The listing builds one solid part. Answer for the finished solid, in the listing's coordinates (mm). Face numbers are marked on the shaded views. A direction names the side the tool comes from. Round coordinates to 2 decimals unless told otherwise and drop trailing zeros. Write each loop counter-clockwise with the first axis right and the second up, starting at its lowest first coordinate (ties: lowest second). Pieces come first, ordered by that corner, then holes.
(1) The mould has two halves that part along Y. Classify the marked faces 1, 2 and 3: +Y half, -Y half, draft (parallel to the pull), parting line (faces both ways), or undercut.
(2) For the marked faces 4, 5, 6, 7 and 8, determine the directions among +Z, -Z, +X, -X, +Y, -Y from which every point of the face is accessible in a straight line to the end or side of a thin tool.
(3) A cutting plane is placed at A-A, the plane y = 46.2. Give the vertices of the cut face in (x, z).
(4) A cutting plane is placed at B-B, the plane y = 12. Give the vertices of the cut face in (x, z).
(5) A cutting plane is placed at C-C, the plane x = 38.5. Give the vertices of the cut face in (y, z), and give its area (3 significant figures).
(6) Find the intervals of material crossed by probe 1 along Y at (x, z) = (34.3, 1.2); probe 2 along Y at (x, z) = (34.5, 15.25); probe 3 along X at (y, z) = (2.5, 5.75), in increasing order.
(7) Each of these flat-tipped pins is pushed along its axis until it touches: pin 1 Ø3 at (y, z) = (30, 8.5) entering from -X; pin 2 Ø2 at (x, z) = (20.5, 9.5) entering from -Y; pin 3 Ø5.5 at (x, y) = (7, 29) entering from +Z. Where does it stop, or does it pass through?
(8) A cutting plane is placed at D-D, the plane y = -3.25. Give the vertices of the cut face in (x, z), and give its area (3 significant figures).
from build123d import *

# Parameters (mm, degrees)
F1_DEPTH = 20
F0_R     = 1.75
F2_DEPTH = 2
F3_DEPTH = 1.3
F4_W     = 13.5
F4_H     = 6.9375
F4_H_2   = 1.25
F4_H_3   = 0.75
F5_DEPTH = 6.1
F6_DEPTH = 13.1
F7_R     = 3


with BuildPart() as f1:
    # F0 (on Top) → F1 (new body)
    with BuildSketch(Plane.XY):
        Polygon((15.3, 50), (15.3, 0), (25.3, 0), (43.3, 0), (53.3, 0), (53.3, 50), (43.3, 50), (25.3, 50), align=None)
    extrude(amount=F1_DEPTH)

    # F0 (on Top) → F2 (join)
    with BuildSketch(Plane.XY):
        with BuildLine():
            Line((43.3, 0), (25.3, 0))
            Line((25.3, 0), (32.379446801, -5.8995390008))
            ThreePointArc((32.379446801, -5.8995390008), (34.3, -6.594875162), (36.220553199, -5.8995390008))
            Line((36.220553199, -5.8995390008), (43.3, 0))
        make_face()
        with Locations((34.3, -3.25)):
            Circle(F0_R, mode=Mode.SUBTRACT)
        with BuildLine():
            Line((32.379446801, 55.8995390008), (25.3, 50))
            Line((25.3, 50), (43.3, 50))
            Line((43.3, 50), (36.220553199, 55.8995390008))
            ThreePointArc((36.220553199, 55.8995390008), (34.3, 56.594875162), (32.379446801, 55.8995390008))
        make_face()
        with Locations((34.3, 53.25)):
            Circle(F0_R, mode=Mode.SUBTRACT)
    extrude(amount=F2_DEPTH)

    # F0 (on Top) → F3 (join)
    with BuildSketch(Plane.XY):
        with BuildLine():
            ThreePointArc((0, 3), (0.8786796564, 0.8786796564), (3, 0))
            Line((3, 0), (15.3, 0))
            Line((15.3, 0), (15.3, 50))
            Line((15.3, 50), (3, 50))
            ThreePointArc((3, 50), (0.8786796564, 49.1213203436), (0, 47))
            Line((0, 47), (0, 3))
        make_face()
        with BuildLine():
            Line((11.0706789419, 2.3), (5.8, 2.3))
            ThreePointArc((5.8, 2.3), (4.3, 3.8), (5.8, 5.3))
            Line((5.8, 5.3), (11.0706789419, 5.3))
            ThreePointArc((11.0706789419, 5.3), (12.5706789419, 3.8), (11.0706789419, 2.3))
        make_face(mode=Mode.SUBTRACT)
        with BuildLine():
            Line((11.0706789419, 44.7), (5.8, 44.7))
            ThreePointArc((5.8, 44.7), (4.3, 46.2), (5.8, 47.7))
            Line((5.8, 47.7), (11.0706789419, 47.7))
            ThreePointArc((11.0706789419, 47.7), (12.5706789419, 46.2), (11.0706789419, 44.7))
        make_face(mode=Mode.SUBTRACT)
    extrude(amount=F3_DEPTH)

    # F4 (on face) → F5 (join)
    with BuildSketch(Plane.XY.offset(1.3)):
        with Locations((8.55, 37.28125)):
            Rectangle(F4_W, F4_H)
        with Locations((8.55, 33.1875)):
            Rectangle(F4_W, F4_H_2)
        with Locations((8.55, 29.09375)):
            Rectangle(F4_W, F4_H)
        Polygon((15.3, 25), (15.3, 25.625), (1.8, 25.625), (1.8, 25), (1.8, 24.375), (15.3, 24.375), align=None)
        with Locations((8.55, 20.90625)):
            Rectangle(F4_W, F4_H)
        with Locations((8.55, 16.8125)):
            Rectangle(F4_W, F4_H_2)
        with Locations((8.55, 12.71875)):
            Rectangle(F4_W, F4_H)
        with Locations((8.55, 8.875)):
            Rectangle(F4_W, F4_H_3)
        with Locations((8.55, 41.125)):
            Rectangle(F4_W, F4_H_3)
    extrude(amount=F5_DEPTH)

    # F4 (on face) → F6 (join)
    with BuildSketch(Plane.XY.offset(1.3)):
        with Locations((8.55, 41.125)):
            Rectangle(F4_W, F4_H_3)
        with Locations((8.55, 8.875)):
            Rectangle(F4_W, F4_H_3)
        with Locations((8.55, 33.1875)):
            Rectangle(F4_W, F4_H_2)
        Polygon((15.3, 25), (15.3, 25.625), (1.8, 25.625), (1.8, 25), (1.8, 24.375), (15.3, 24.375), align=None)
        with Locations((8.55, 16.8125)):
            Rectangle(F4_W, F4_H_2)
    extrude(amount=F6_DEPTH)

    # F7
    f7_edges = [f1.edges().sort_by_distance(p)[0] for p in [
        (1.8, 41.125, 14.4),
        (1.8, 33.1875, 14.4),
        (1.8, 8.875, 14.4),
        (1.8, 25, 14.4),
        (1.8, 16.8125, 14.4),
    ]]
    fillet(f7_edges, radius=F7_R)


solid = f1.part
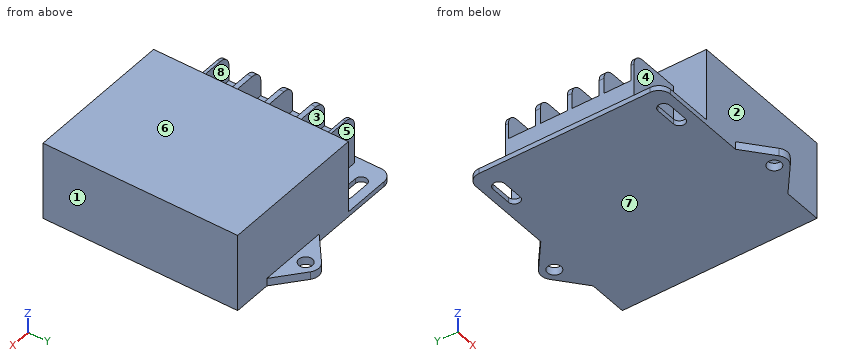
Solutions:
1. face 1: draft
1. face 2: -Y half
1. face 3: undercut
2. face 4: +Z, -X, -Y
2. face 5: +Z, -X, +Y
2. face 6: +Z, +X, -X, +Y, -Y
2. face 7: -Z, +X, -X, +Y, -Y
2. face 8: +Z, -X
3. outline: (0, 0) - (4.3, 0) - (4.3, 1.3) - (0, 1.3) - close; (12.57, 0) - (53.3, 0) - (53.3, 20) - (15.3, 20) - (15.3, 1.3) - (12.57, 1.3) - close
4. outline: (0, 0) - (53.3, 0) - (53.3, 20) - (15.3, 20) - (15.3, 7.4) - (1.8, 7.4) - (1.8, 1.3) - (0, 1.3) - close
5. outline: (-4, 0) - (54, 0) - (54, 2) - (50, 2) - (50, 20) - (0, 20) - (0, 2) - (-4, 2) - close
5. area: 1,020 mm2
6. probe 1: y = -6.59 to -5, -1.5 to 51.5, 55 to 56.59
6. probe 2: y = 0 to 50
6. probe 3: x = 15.3 to 53.3
7. pin 1: stops at x = 1.8
7. pin 2: stops at y = 0
7. pin 3: stops at z = 7.4
8. outline: (29.2, 0) - (32.55, 0) - (32.55, 2) - (29.2, 2) - close; (36.05, 0) - (39.4, 0) - (39.4, 2) - (36.05, 2) - close
8. area: 13.4 mm2
